Check sheet for the modelled part. Datum: model origin and axes. Units: mm. A direction names the side the tool comes from. Round coordinates to 2 decimals unless told otherwise and drop trailing zeros. Write each loop counter-clockwise with the first axis right and the second up, starting at its lowest first coordinate (ties: lowest second). Pieces come first, ordered by that corner, then holes. Notation, with made-up numbers: M 29,-28 L 35,-28 A33 cw 35,5 Z; hole C 49.25,54.5 d9. An arc over 180 degrees is marked long. Answer in a Markdown table with one row per item.
```python
from build123d import *

# Parameters (mm, degrees)
BOSS_EXTRU_1_DEPTH           = 1.5
ESQUISSE2_R                  = 1.5
ENL_V_MAT_EXTRU_1_DEPTH      = 10
ESQUISSE3_W                  = 260.587519956
ESQUISSE3_H                  = 19.442661658
ENL_V_MAT_EXTRU_2_DEPTH      = 230.841793415
CONG_1_R                     = 10
CONG_2_R                     = 1
ESQUISSE4_R                  = 1.5
ENL_V_MAT_EXTRU_3_DEPTH      = 230.841793557
R_P_TITION_CIRCULAIRE1_COUNT = 3
R_P_TITION_CIRCULAIRE1_ANGLE = 180
ESQUISSE5_R                  = 1.5
ENL_V_MAT_EXTRU_4_DEPTH      = 230.841793557
ENL_V_MAT_EXTRU_5_DEPTH      = 230.841793557
ENL_V_MAT_EXTRU_6_DEPTH      = 225.685335667
CONG_3_R                     = 3
ESQUISSE8_R                  = 1.25
ENL_V_MAT_EXTRU_7_DEPTH      = 4
ENL_V_MAT_EXTRU_8_DEPTH      = 225.685335667
CONG_4_R                     = 3


with BuildPart() as part:
    # Esquisse1 → Boss.-Extru.1 (new body)
    with BuildSketch(Plane(origin=(0, 0, 0), x_dir=(1, 0, 0), z_dir=(0, 1, 0))):
        with BuildLine():
            Line((165, -54.556978373), (165, 55.241669751))
            Line((165, 55.241669751), (104.517749831, 160))
            Line((104.517749831, 160), (-104.517749831, 160))
            Line((-104.517749831, 160), (-165, 55.241669751))
            Line((-165, 55.241669751), (-165, -54.556978373))
            ThreePointArc((-165, -54.556978373), (-144.278322914, -96.877393783), (-112.949332972, -132.075402973))
            ThreePointArc((-112.949332972, -132.075402973), (0, -145), (112.949332972, -132.075402973))
            ThreePointArc((112.949332972, -132.075402973), (144.278322914, -96.877393783), (165, -54.556978373))
        make_face()
    extrude(amount=BOSS_EXTRU_1_DEPTH)

    # Esquisse2 → Enlèv. mat.-Extru.1 (cut)
    with BuildSketch(Plane(origin=(0, 1.5, 0), x_dir=(1, 0, 0), z_dir=(0, 1, 0))):
        with Locations(Location((-106.773123959, -106.773123959, 0), (0, 0, 270))):
            Circle(ESQUISSE2_R)
        with Locations(Location((143, -86.912961133, 0), (0, 0, 270))):
            Circle(ESQUISSE2_R)
        with Locations(Location((133.434799764, -83.996294466, 0), (0, 0, 270))):
            Circle(ESQUISSE2_R)
        with Locations(Location((147.434799764, -38.083333333, 0), (0, 0, 270))):
            Circle(ESQUISSE2_R)
        with Locations(Location((157, -41, 0), (0, 0, 270))):
            Circle(ESQUISSE2_R)
        with Locations(Location((-147.434799764, -38.083333333, 0), (0, 0, 270))):
            Circle(ESQUISSE2_R)
        with Locations(Location((-157, -41, 0), (0, 0, 270))):
            Circle(ESQUISSE2_R)
        with Locations(Location((-143, -86.912961133, 0), (0, 0, 270))):
            Circle(ESQUISSE2_R)
        with Locations(Location((-133.434799764, -83.996294466, 0), (0, 0, 270))):
            Circle(ESQUISSE2_R)
        with Locations(Location((106.773123959, -106.773123959, 0), (0, 0, 270))):
            Circle(ESQUISSE2_R)
        with BuildLine():
            Line((-92.34673338, -78.53312836), (-104.066636173, -145))
            Line((-104.066636173, -145), (104.066636173, -145))
            Line((104.066636173, -145), (92.34673338, -78.53312836))
            ThreePointArc((92.34673338, -78.53312836), (77.639867217, -53.060088946), (50, -43))
            Line((50, -43), (-50, -43))
            ThreePointArc((-50, -43), (-77.639867217, -53.060088946), (-92.34673338, -78.53312836))
        make_face()
        Polygon((141.485532979, -40.451080094), (166.980337187, -48.225077896), (155.31367052, -86.48587884), (129.818866313, -78.711881039), align=None)
        Polygon((-141.485532979, -40.451080094), (-166.980337187, -48.225077896), (-155.31367052, -86.48587884), (-129.818866313, -78.711881039), align=None)
        with BuildLine():
            ThreePointArc((18.81620543, -19.363636364), (0, -3), (-18.81620543, -19.363636364))
            ThreePointArc((-18.81620543, -19.363636364), (0, 27), (18.81620543, -19.363636364))
        make_face()
    extrude(amount=-ENL_V_MAT_EXTRU_1_DEPTH, mode=Mode.SUBTRACT)

    # Esquisse3 → Enlèv. mat.-Extru.2 (cut, through all)
    with BuildSketch(Plane(origin=(0, 1.5, 0), x_dir=(1, 0, 0), z_dir=(0, 1, 0))):
        with Locations((0, -124.721330829)):
            Rectangle(ESQUISSE3_W, ESQUISSE3_H)
    extrude(amount=-ENL_V_MAT_EXTRU_2_DEPTH, mode=Mode.SUBTRACT)

    # Congé1
    cong_1_edges = [part.edges().sort_by_distance(p)[0] for p in [
        (-165, 0.75, -55.241669751),
        (-104.517749831, 0.75, -160),
        (104.517749831, 0.75, -160),
        (165, 0.75, -55.241669751),
        (98.776826752, 0.75, 115),
        (-98.776826752, 0.75, 115),
        (-130.293759978, 0.75, 115),
        (130.293759978, 0.75, 115),
    ]]
    fillet(cong_1_edges, radius=CONG_1_R)

    # Congé2
    cong_2_edges = [part.edges().sort_by_distance(p)[0] for p in [
        (-18.81620543, 0.75, 19.363636364),
        (18.81620543, 0.75, 19.363636364),
    ]]
    fillet(cong_2_edges, radius=CONG_2_R)

    # Esquisse4 → Enlèv. mat.-Extru.3 (cut, through all)
    with BuildSketch(Plane(origin=(0, 1.5, 0), x_dir=(1, 0, 0), z_dir=(0, 1, 0))):
        with Locations(Location((-124.54257934, -80.8788967, 0), (0, 0, 270))):
            Circle(ESQUISSE4_R)
        with Locations(Location((-145.771636742, -28.335135813, 0), (0, 0, 270))):
            Circle(ESQUISSE4_R)
        with Locations(Location((-145.771636742, 28.335135813, 0), (0, 0, 270))):
            Circle(ESQUISSE4_R)
        with Locations(Location((-124.54257934, 80.8788967, 0), (0, 0, 270))):
            Circle(ESQUISSE4_R)
    enl_v_mat_extru_3 = extrude(amount=-ENL_V_MAT_EXTRU_3_DEPTH, mode=Mode.SUBTRACT)

    # Répétition circulaire1: Enlèv. mat.-Extru.3 ×3 about axis
    r_p_tition_circulaire1_axis = Axis((0, 0, 0), (0, -1, 0))
    for i in range(1, R_P_TITION_CIRCULAIRE1_COUNT):
        add(enl_v_mat_extru_3.rotate(r_p_tition_circulaire1_axis, i * R_P_TITION_CIRCULAIRE1_ANGLE / (R_P_TITION_CIRCULAIRE1_COUNT - 1)), mode=Mode.SUBTRACT)

    # Esquisse5 → Enlèv. mat.-Extru.4 (cut, through all)
    with BuildSketch(Plane(origin=(0, 1.5, 0), x_dir=(1, 0, 0), z_dir=(0, 1, 0))):
        with Locations(Location((-70, -40, 0), (0, 0, 270))):
            Circle(ESQUISSE5_R)
        with Locations(Location((70, -40, 0), (0, 0, 90))):
            Circle(ESQUISSE5_R)
    extrude(amount=-ENL_V_MAT_EXTRU_4_DEPTH, mode=Mode.SUBTRACT)

    # Esquisse6 → Enlèv. mat.-Extru.5 (cut, through all)
    with BuildSketch(Plane(origin=(0, 1.5, 0), x_dir=(1, 0, 0), z_dir=(0, 1, 0))):
        with BuildLine():
            Line((-165, 40), (-147.160626528, 40))
            ThreePointArc((-147.160626528, 40), (0, 152.5), (147.160626528, 40))
            Line((147.160626528, 40), (165, 40))
            Line((165, 40), (165, 160))
            Line((165, 160), (-165, 160))
            Line((-165, 160), (-165, 40))
        make_face()
    extrude(amount=-ENL_V_MAT_EXTRU_5_DEPTH, mode=Mode.SUBTRACT)

    # Esquisse7 → Enlèv. mat.-Extru.6 (cut, through all)
    with BuildSketch(Plane(origin=(0, 1.5, 0), x_dir=(1, 0, 0), z_dir=(0, 1, 0))):
        Polygon((126.695788782, 122.365900164), (126.695788782, 84.8788967), (112.653221515, 84.8788967), (91.010089974, 122.365900164), align=None)
        Polygon((-91.010089974, 122.365900164), (-112.653221515, 84.8788967), (-126.695788782, 84.8788967), (-126.695788782, 122.365900164), align=None)
    extrude(amount=-ENL_V_MAT_EXTRU_6_DEPTH, mode=Mode.SUBTRACT)

    # Congé3
    cong_3_edges = [part.edges().sort_by_distance(p)[0] for p in [
        (-151.413225219, 0.75, 85.296536378),
        (-165, 0.75, 47.621223996),
        (-165, 0.75, -40),
        (165, 0.75, -40),
        (147.160626528, 0.75, -40),
        (-147.160626528, 0.75, -40),
        (91.010089974, 0.75, -122.365900164),
        (126.695788782, 0.75, -84.8788967),
        (112.653221515, 0.75, -84.8788967),
        (-91.010089974, 0.75, -122.365900164),
        (-112.653221515, 0.75, -84.8788967),
        (-126.695788782, 0.75, -84.8788967),
        (165, 0.75, 47.621223996),
        (151.413225219, 0.75, 85.296536378),
    ]]
    fillet(cong_3_edges, radius=CONG_3_R)

    # Esquisse8 → Enlèv. mat.-Extru.7 (cut)
    with BuildSketch(Plane(origin=(0, 1.5, 0), x_dir=(1, 0, 0), z_dir=(0, 1, 0))):
        with Locations(Location((-35, 0, 0), (0, 0, 270))):
            Circle(ESQUISSE8_R)
        with Locations(Location((-35, 10, 0), (0, 0, 270))):
            Circle(ESQUISSE8_R)
        with Locations(Location((0, 30, 0), (0, 0, 270))):
            Circle(ESQUISSE8_R)
        with Locations(Location((25.980762114, -15, 0), (0, 0, 270))):
            Circle(ESQUISSE8_R)
        with Locations(Location((-25.980762114, -15, 0), (0, 0, 270))):
            Circle(ESQUISSE8_R)
    extrude(amount=-ENL_V_MAT_EXTRU_7_DEPTH, mode=Mode.SUBTRACT)

    # Esquisse9 → Enlèv. mat.-Extru.8 (cut, through all)
    with BuildSketch(Plane(origin=(0, 1.5, 0), x_dir=(1, 0, 0), z_dir=(0, 1, 0))):
        Polygon((-25, 152.5), (25, 152.5), (23.278688525, 142), (-23.278688525, 142), align=None)
    extrude(amount=-ENL_V_MAT_EXTRU_8_DEPTH, mode=Mode.SUBTRACT)

    # Congé4
    cong_4_edges = [part.edges().sort_by_distance(p)[0] for p in [
        (-24.670691628, 0.75, -150.491218929),
        (-23.278688525, 0.75, -142),
        (24.670691628, 0.75, -150.491218929),
        (23.278688525, 0.75, -142),
    ]]
    fillet(cong_4_edges, radius=CONG_4_R)


solid = part.part
```
1. Section check D-D, the plane z = -116.5. Record the cut outline in (x, y), and give its area (3 significant figures).
Found:
| item | result |
|---|---|
| outline | M -94.4,0 L 94.4,0 L 94.4,1.5 L -94.4,1.5 Z |
| area | 283 mm2 |
2. Section check A-A, the plane x = -6. Record the cut outline in (y, z), and give its area (3 significant figures).
Found:
| item | result |
|---|---|
| outline | M 0,-142 L 1.5,-142 L 1.5,-26.32 L 0,-26.32 Z; M 0,3.97 L 1.5,3.97 L 1.5,43 L 0,43 Z |
| area | 232 mm2 |
3. Section check C-C, the plane y = 1.1. Count the separate pieces of the cut face and the enclosed holes in it, and give its area (3 significant figures).
Found:
| item | result |
|---|---|
| separate pieces | 1 |
| enclosed holes | 30 |
| area | 56,000 mm2 |
4. Scan lines: L1, parallel to X at y = 0.65, z = -13; L2, parallel to Z at x = -29, y = 0.4; L3, parallel to Z at x = 118, y = 0.1. Record each from-to range of solid material in increasing order.
Found:
| item | result |
|---|---|
| L1 | x = -165 to -23.66, 23.66 to 165 |
| L2 | z = -149.72 to -147.12, -144.43 to 43 |
| L3 | z = -84.88 to 115 |
5. Access from +Z, -Z, +X, -X, +Y, -Y to the whole of each face (thin tool, end or side, straight path). Record for faces 4 (the face through (0, 1, 3)), 5 (the face through (138.49, 0.76, -63.85)), 6 (the face through (77.96, 0.76, 53.33)).
Found:
| item | result |
|---|---|
| face 4 | +Y, -Y |
| face 5 | -Z, +X, +Y, -Y |
| face 6 | +Z, +Y, -Y |
6. Section check B-B, the plane z = 96.5. Record the cut outline in (x, y), and give its area (3 significant figures).
Found:
| item | result |
|---|---|
| outline | M -144.53,0 L -95.51,0 L -95.51,1.5 L -144.53,1.5 Z; M 95.51,0 L 144.53,0 L 144.53,1.5 L 95.51,1.5 Z |
| area | 147 mm2 |
7. Draft check along Z on faces 1 (the face through (-77.317, 0.76, 52.792)), 2 (the face through (-61.09, 0.76, -139.73)), 3 (the face through (135.57, 0.76, 59.85)). Enter one of: +Z half, -Z half, draft (parallel to the pull), parting line (faces both ways), or undercut.
Found:
| item | result |
|---|---|
| face 1 | +Z half |
| face 2 | -Z half |
| face 3 | undercut |
